Design review of the part built by this model. Coordinates are the model's own, in mm. A direction names the side the tool comes from. Give positions to 0.01 mm unless a question says otherwise; leave off trailing zeros. Write each loop counter-clockwise with the first axis right and the second up, starting at its lowest first coordinate (ties: lowest second). Pieces come first, ordered by that corner, then holes. Notation, with made-up numbers: (34.5, 70.5) -> (38.5, 70.5) arc R15 cw to (38.5, 97.5) -> close; hole circle Ø4 at (1, 32). An arc over 180 degrees is marked (long way). Write each question's results on one line, items separated by ' | '. Start each with the question number.
(1) Take a section at B-B (z = 0). State the section outline as (x, y) points (3 decimals), plus the area to 3 significant figures.
(2) Take a section at D-D (z = 4.5). State the section outline as (x, y) points.
(3) Take a section at A-A (x = 0). State the section outline as (y, z) points (3 decimals), plus the area to 3 significant figures.
(4) To check wall thickness, follow probe 1 along Z at (x, y) = (0, 50) (3 decimals); probe 2 along Z at (x, y) = (0, 54.5); probe 3 along Z at (x, y) = (1, 13). State the ranges of each line that lie inside material, in increasing order.
(5) For faces 1 (the face through (0, 18, 8.65)), 2 (the face through (4, 52.101, 0)), 3 (the face through (-14.14, 48.2, -0.01)), 4 (the face through (14.1, 24.8, 9.51)), 5 (the face through (0, 25, 15)), list the 3-axis set-ups (+Z, -Z, +X, -X, +Y, -Y) from which the entire face can be reached by the end or side of a thin tool; tool diameter is ignored.
(6) Clearance check with flat-ended pins moving along their axes: pin 1 (8 mm diameter, centred on x = 3, y = 11.5, fed in from -Z); pin 2 (8 mm diameter, centred on x = 10, y = 48.5, fed in from -Z); pin 3 (8 mm diameter, centred on x = 7.5, z = 10, fed in from -Y); pin 4 (12 mm diameter, centred on x = 8.5, z = 4.5, fed in from -Y). State where each tip first meets the part, or that it passes through.
(7) Mouldability with a two-part tool opening along X and no side actions: class faces 6 (the face through (0, 47.3, -9)), 7 (the face through (-14.1, 25.5, 9.51)), 8 (the face through (0, 3, 12)) as released by +X, released by -X, zero draft, split by the parting line, or undercut.
(8) Take a section at C-C (y = 9.5). State the section outline as (x, z) points, plus the area to 3 significant figures.
Autodesk Inventor part; units mm, degrees
ref_plane "YZ Plane" through (0, 0, 0) normal (1, 0, 0) x (0, 1, 0)
ref_plane "XZ Plane" through (0, 0, 0) normal (0, 1, 0) x (-1, 0, 0)
ref_plane "XY Plane" through (0, 0, 0) normal (0, 0, 1) x (1, 0, 0)
sketch "Sketch1" plane through (0, 0, 0) normal (0, 0, 1) x (1, 0, 0)
  arc A0 (-15, 0) -> (15, 0) centre (0, 0) ccw
  line L0 (-15, 60) -> (15, 60)
  line L1 (15, 60) -> (15, 0)
  line L2 (-15, 0) -> (-15, 60)
  dimension "d0" = 30
  dimension "d1" = 60
extrude "Extrusion1" add sketch "Sketch1" along normal mid plane 30
sketch "Sketch2" plane through (0, 0, -15) normal (0, 0, -1) x (-1, 0, 0)
  arc A0 (-15, 0) -> (15, 0) centre (0, 0) ccw
  line L0 (15, 0) -> (15, 47.3)
  line L1 (15, 47.3) -> (-15, 47.3)
  line L2 (-15, 47.3) -> (-15, 0)
  line L3 (15, 0) -> (15, 60)
  line L4 (-15, 60) -> (-15, 0)
  line L5 (15, 60) -> (-15, 60)
  dimension "d4" = 12.7
extrude "Extrusion2" cut sketch "Sketch2" against normal blind 23.65 contours L2 L1 L0 A0
fillet "Fillet1" radius 3 11 edges at (-15, 53.65, -15) (15, 53.65, -15) (0, -15, 15) (15, 30, 15) (-15, 30, 15) (0, -15, 8.65) (15, 23.65, 8.65) (-15, 23.65, 8.65) (-15, 47.3, -3.175) (0, 47.3, -15) (15, 47.3, -3.175)
sketch "Sketch3" plane through (-12, 47.3, -15) normal (0, -1, 0) x (1, 0, 0)
  point P0 (12, 15)
  point P1 (12, 15)
hole "Hole1" at (0, 47.3, 0) direction (0, 1, 0) diameter 6.604 end through all counterbore diameter 16.51 counterbore depth 4.8006
sketch "Sketch4" plane through (0, 0, 15) normal (0, 0, 1) x (1, 0, 0)
  point P0 (0, 0)
  point P1 (0, 0)
hole "Hole2" at (0, 0, 15) direction (0, 0, -1) diameter 6 end through all
properties part number "NASA-20-ARM-HG-01"
Report:
1) outline: (-15, 50.3) arc R3 ccw to (-12, 47.3) -> (-8.255, 47.3) -> (-8.255, 52.101) -> (-3.302, 52.101) -> (-3.302, 60) -> (-15, 60) -> close; (3.302, 52.101) -> (8.255, 52.101) -> (8.255, 47.3) -> (12, 47.3) arc R3 ccw to (15, 50.3) -> (15, 60) -> (3.302, 60) -> close | area: 246 mm2
2) outline: (-15, 50.3) arc R3 ccw to (-12, 47.3) -> (-6.92, 47.3) -> (-6.92, 52.1) -> (6.92, 52.1) -> (6.92, 47.3) -> (12, 47.3) arc R3 ccw to (15, 50.3) -> (15, 60) -> (-15, 60) -> close
3) outline: (-15, 11.65) arc R3 ccw to (-12, 8.65) -> (-3, 8.65) -> (-3, 15) -> (-12, 15) arc R3 ccw to (-15, 12) -> close; (3, 8.65) -> (47.3, 8.65) -> (47.3, 8.255) -> (52.101, 8.255) -> (52.101, 3.302) -> (60, 3.302) -> (60, 15) -> (3, 15) -> close; (47.3, -12) arc R3 ccw to (50.3, -15) -> (60, -15) -> (60, -3.302) -> (52.101, -3.302) -> (52.101, -8.255) -> (47.3, -8.255) -> close | area: 601 mm2
4) probe 1: -14.985 to -8.255, 8.255 to 15 | probe 2: -15 to -3.3, 3.3 to 15 | probe 3: 8.65 to 15
5) face 1: -Z, +X, -X, -Y | face 2: -Y | face 3: -Z, -X, -Y | face 4: -Z, +X, -Y | face 5: +Z, +X, -X, +Y, -Y
6) pin 1: z = 8.65 | pin 2: z = -15 | pin 3: y = -14.51 | pin 4: y = -13.19
7) face 6: zero draft | face 7: released by -X | face 8: undercut
8) outline: (-15, 11.65) arc R3 ccw to (-12, 8.65) -> (12, 8.65) arc R3 ccw to (15, 11.65) -> (15, 12) arc R3 ccw to (12, 15) -> (-12, 15) arc R3 ccw to (-15, 12) -> close | area: 183 mm2
